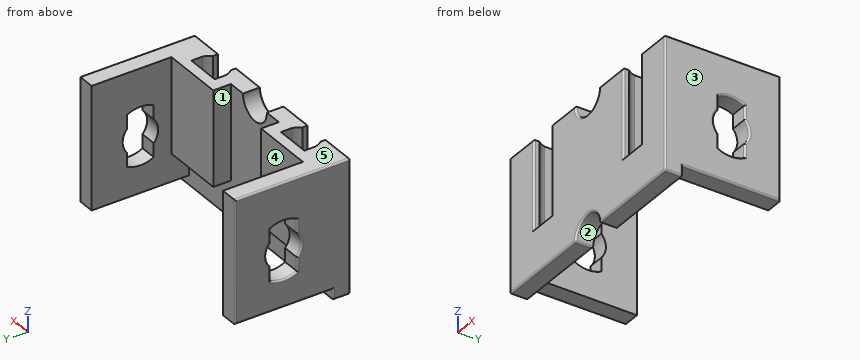
```python
from build123d import *

# Parameters (mm, degrees)
SKETCH_1_W          = 26
SKETCH_1_H          = 15
EXTRUDE_1_DEPTH     = 2
SKETCH_2_W          = 2
SKETCH_2_H          = 13.8
EXTRUDE_2_DEPTH     = 11
SKETCH_3_W          = 7
SKETCH_3_H          = 10.7
EXTRUDE_3_DEPTH     = 2
CUT_EXTRUDE_1_REACH = 32.021
CUT_EXTRUDE_2_DEPTH = 10
CUT_EXTRUDE_3_REACH = 20.608
SKETCH_6_R          = 2
FILLET_1_R          = 0.2


with BuildPart() as part:
    # 草图1 → 凸台-拉伸1 (new body)
    with BuildSketch(Plane(origin=(0, 0, 0), x_dir=(1, 0, 0), z_dir=(0, 1, 0))):
        Rectangle(SKETCH_1_W, SKETCH_1_H)
    extrude(amount=EXTRUDE_1_DEPTH)

    # 草图2 → 凸台-拉伸2 (add)
    with BuildSketch(Plane(origin=(0, 2, 0), x_dir=(1, 0, 0), z_dir=(0, 1, 0))):
        with Locations((-12, -0.6)):
            Rectangle(SKETCH_2_W, SKETCH_2_H)
    extrude_2 = extrude(amount=EXTRUDE_2_DEPTH)

    # 草图3 → 凸台-拉伸3 (add)
    with BuildSketch(Plane(origin=(0, 2, 0), x_dir=(1, 0, 0), z_dir=(0, 1, 0))):
        with Locations((-7.5, -2.15)):
            Rectangle(SKETCH_3_W, SKETCH_3_H)
    extrude_3 = extrude(amount=EXTRUDE_3_DEPTH)

    # 草图4 → 切除-拉伸1 (cut, up to next)
    with BuildSketch(Plane.ZY.offset(13), mode=Mode.PRIVATE) as cut_extrude_1_sk1:
        with BuildLine():
            Line((-2.883140649, 6), (-1.322875656, 6))
            ThreePointArc((-1.322875656, 6), (0, 5.5), (1.322875656, 6))
            Line((1.322875656, 6), (2.883140649, 6))
            ThreePointArc((2.883140649, 6), (3.25, 7.5), (2.883140649, 9))
            Line((2.883140649, 9), (1.322875656, 9))
            ThreePointArc((1.322875656, 9), (0, 9.5), (-1.322875656, 9))
            Line((-1.322875656, 9), (-2.883140649, 9))
            ThreePointArc((-2.883140649, 9), (-3.25, 7.5), (-2.883140649, 6))
        make_face()
    cut_extrude_1_tool1 = extrude(cut_extrude_1_sk1.sketch, amount=-CUT_EXTRUDE_1_REACH, mode=Mode.PRIVATE) & part.part
    cut_extrude_1 = cut_extrude_1_tool1.solids().sort_by_distance((-13, 7.5, 0))[0]
    add(cut_extrude_1, mode=Mode.SUBTRACT)

    # 草图5 → 切除-拉伸2 (cut)
    with BuildSketch(Plane.XY.offset(7.5)):
        with BuildLine():
            Line((-6, 0), (-9, 0))
            Line((-9, 0), (-9, 0.677124344))
            ThreePointArc((-9, 0.677124344), (-9.280042303, 1.088161527), (-9.45, 1.555590279))
            Line((-9.45, 1.555590279), (-9.45, 2.8))
            Line((-9.45, 2.8), (-5.55, 2.8))
            Line((-5.55, 2.8), (-5.55, 1.555590279))
            ThreePointArc((-5.55, 1.555590279), (-5.719957697, 1.088161527), (-6, 0.677124344))
            Line((-6, 0.677124344), (-6, 0))
        make_face()
    cut_extrude_2 = extrude(amount=-CUT_EXTRUDE_2_DEPTH, mode=Mode.SUBTRACT)

    # 镜向1: 凸台-拉伸2, 凸台-拉伸3, 切除-拉伸1, 切除-拉伸2 across plane
    add(extrude_2.mirror(Plane(origin=(0, 0, 0), x_dir=(0, 0, 1), z_dir=(1, 0, 0))))
    add(extrude_3.mirror(Plane(origin=(0, 0, 0), x_dir=(0, 0, 1), z_dir=(1, 0, 0))))
    add(cut_extrude_1.mirror(Plane(origin=(0, 0, 0), x_dir=(0, 0, 1), z_dir=(1, 0, 0))), mode=Mode.SUBTRACT)
    add(cut_extrude_2.mirror(Plane(origin=(0, 0, 0), x_dir=(0, 0, 1), z_dir=(1, 0, 0))), mode=Mode.SUBTRACT)

    # 草图6 → 切除-拉伸3 (cut, up to next)
    with BuildSketch(Plane(origin=(0, 2, 0), x_dir=(1, 0, 0), z_dir=(0, 1, 0)), mode=Mode.PRIVATE) as cut_extrude_3_sk1:
        with Locations((0, -7.5)):
            Circle(SKETCH_6_R)
    cut_extrude_3_tool1 = extrude(cut_extrude_3_sk1.sketch, amount=-CUT_EXTRUDE_3_REACH, mode=Mode.PRIVATE) & part.part
    # 草图6 → 切除-拉伸3 (cut, up to next)
    with BuildSketch(Plane(origin=(0, 2, 0), x_dir=(1, 0, 0), z_dir=(0, 1, 0)), mode=Mode.PRIVATE) as cut_extrude_3_sk2:
        with Locations((0, 7.5)):
            Circle(SKETCH_6_R)
    cut_extrude_3_tool2 = extrude(cut_extrude_3_sk2.sketch, amount=-CUT_EXTRUDE_3_REACH, mode=Mode.PRIVATE) & part.part
    add(cut_extrude_3_tool1.solids().sort_by_distance((0, 2, 7.5))[0], mode=Mode.SUBTRACT)
    add(cut_extrude_3_tool2.solids().sort_by_distance((0, 2, -7.5))[0], mode=Mode.SUBTRACT)

    # 圆角1
    fillet_1_edges = [part.edges().sort_by_distance(p)[0] for p in [
        (13, 5.5, 0),
        (13, 6, 2.103008152),
        (13, 7.5, 3.25),
        (13, 9, 2.103008152),
        (13, 9.5, 0),
        (13, 9, -2.103008152),
        (13, 7.5, -3.25),
        (13, 6, -2.103008152),
        (11, 0, 7.5),
        (6, 0, 2.5),
        (9, 0, 2.5),
        (7.5, 0, -2.5),
        (-13, 7.5, -6.3),
        (4, 0, 7.5),
        (0, 0, 5.5),
        (-13, 13, 0.6),
        (-7.5, 0, -7.5),
        (-7.5, 2, -7.5),
        (2, 1, -7.5),
        (-2, 1, -7.5),
        (0, 0, -5.5),
        (7.5, 2, -7.5),
        (13, 0, 0),
        (-11, 0, 7.5),
        (-13, 5.5, 0),
        (-13, 6, 2.103008152),
        (-13, 7.5, 3.25),
        (-13, 9, 2.103008152),
        (-13, 9.5, 0),
        (-13, 9, -2.103008152),
        (-13, 7.5, -3.25),
        (-13, 6, -2.103008152),
        (-13, 0, 0),
        (7.5, 0, -7.5),
        (-4, 0, 7.5),
        (-13, 2, -6.9),
        (13, 1, -7.5),
        (-7.5, 0, -2.5),
        (-6, 0, 2.5),
        (-9, 0, 2.5),
        (13, 6.5, 7.5),
        (-13, 6.5, 7.5),
        (-13, 1, -7.5),
        (13, 2, -6.9),
        (13, 13, 0.6),
        (13, 7.5, -6.3),
    ]]
    fillet(fillet_1_edges, radius=FILLET_1_R)


solid = part.part
```
Work out the finished part from the listing and answer in its coordinate system (mm). Face numbers are marked on the shaded views. A direction names the side the tool comes from. Coordinates: 2 decimals unless noted, no trailing zeros. Loops run counter-clockwise (first coordinate to the right, second up) from the corner with the lowest first, then second, coordinate; pieces in that order, holes last. Notation, with made-up numbers: M -26.75,-27.75 L -7.75,-27.75 A27 cw -7.75,-4.75 Z; hole C 29.5,36.5 d3. An arc over 180 degrees is marked long. Use CSV: the item, a comma, the result in double quotes. Start each with the question number.
(1) Given pin 1 Ø2 at (x, z) = (0, -4.5) entering from +Y; pin 2 Ø1.5 at (x, y) = (0, 3.5) entering from +Z; pin 3 Ø6 at (x, z) = (5.5, 3) entering from +Y; pin 4 Ø2 at (x, y) = (-7, 1) entering from +Z, each flat-ended and moving along its own axis, determine where each tip first touches the part or whether it passes through.
(2) Find section C-C, the plane x = 4.5. Give the vertices of the cut face in (y, z), then the cut area to 3 significant figures.
(3) Find section D-D, the plane y = 12.25. Give the vertices of the cut face in (x, z), then the cut area to 3 significant figures.
(4) For the marked faces 1 and 2, determine the directions among +Z, -Z, +X, -X, +Y, -Y from which every point of the face is accessible in a straight line to the end or side of a thin tool.
(5) Consider line 1 (X direction, y = 2.5, z = 4.25); line 2 (X direction, y = 8, z = -5.5); line 3 (X direction, y = 3.25, z = 1). Determine where each line is inside the solid, lowest interval first.
(6) For a pull along X with two mould halves and no side action, classify the marked faces 3, 4 and 5 as +X half, -X half, draft (parallel to the pull), parting line (faces both ways), or undercut.
(7) Find section B-B, the plane y = 7.5. Give the vertices of the cut face in (x, z), then the cut area to 3 significant figures.
(8) Find section A-A, the plane y = 3.25. Give the vertices of the cut face in (x, z).
Recorded:
1,pin 1,"stops at y = 2"
1,pin 2,"passes through"
1,pin 3,"stops at y = 4"
1,pin 4,"stops at z = -2.5"
2,outline,"M 0,-7.3 A0.2 ccw 0.2,-7.5 L 1.8,-7.5 A0.2 ccw 2,-7.3 L 2,-3.2 L 4,-3.2 L 4,7.5 L 0.2,7.5 A0.2 ccw 0,7.3 Z"
2,area,"51.4 mm^2"
3,outline,"M -13,-6.1 A0.2 ccw -12.8,-6.3 L -11,-6.3 L -11,7.5 L -12.8,7.5 A0.2 ccw -13,7.3 Z; M 11,-6.3 L 12.8,-6.3 A0.2 ccw 13,-6.1 L 13,7.3 A0.2 ccw 12.8,7.5 L 11,7.5 Z"
3,area,"55.2 mm^2"
4,face 1,"+Z, -Z, +Y"
4,face 2,"-Z, +Y, -Y"
5,line 1,"x = -13 to -9.45, -5.55 to -4, 4 to 5.55, 9.45 to 13"
5,line 2,"x = -13 to -11, 11 to 13"
5,line 3,"x = -13 to -4, 4 to 13"
6,face 3,"+X half"
6,face 4,"undercut"
6,face 5,"draft"
7,outline,"M -13,-6.1 A0.2 ccw -12.8,-6.3 L -11,-6.3 L -11,-3.25 L -12.8,-3.25 A0.2 ccw -13,-3.45 Z; M -13,3.45 A0.2 ccw -12.8,3.25 L -11,3.25 L -11,7.5 L -12.8,7.5 A0.2 ccw -13,7.3 Z; M 11,-6.3 L 12.8,-6.3 A0.2 ccw 13,-6.1 L 13,-3.45 A0.2 ccw 12.8,-3.25 L 11,-3.25 Z; M 11,3.25 L 12.8,3.25 A0.2 ccw 13,3.45 L 13,7.3 A0.2 ccw 12.8,7.5 L 11,7.5 Z"
7,area,"29.1 mm^2"
8,outline,"M -13,-6.1 A0.2 ccw -12.8,-6.3 L -11,-6.3 L -11,-3.2 L -4,-3.2 L -4,7.5 L -12.8,7.5 A0.2 ccw -13,7.3 Z; M 4,-3.2 L 11,-3.2 L 11,-6.3 L 12.8,-6.3 A0.2 ccw 13,-6.1 L 13,7.3 A0.2 ccw 12.8,7.5 L 4,7.5 Z"
